Can you work these out from the drawing? Everything is in mm from the part's minimum corner. A direction names the side the tool comes from. Coordinates: 2 decimals unless noted, no trailing zeros. Order: outer loops, then holes, each group sorted by start corner. A loop starts at its lowest first (then second) coordinate and runs counter-clockwise, first axis right, second up. Notation, with made-up numbers: (30.5, -2) -> (48.5, -2) arc R6 cw to (48.5, 4) -> close; hole circle Ø10 at (-8.5, 67). An arc over 180 degrees is marked (long way). Answer in a Markdown table with one row per item.
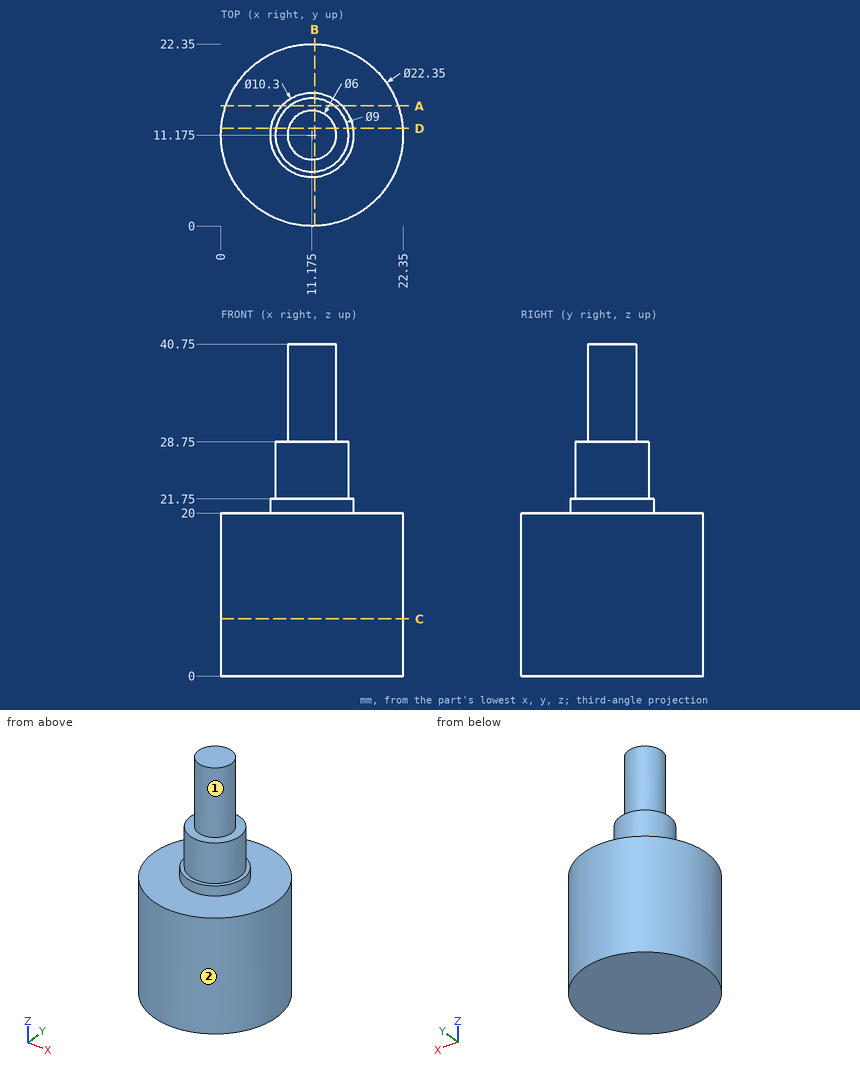
(1) Suppose I cut it at C-C (z = 7). Please give me the cut outline in (x, y) (3 decimals), and give its area (3 significant figures).
Response values:
| item | result |
|---|---|
| outline | circle Ø22.35 at (11.175, 11.175) |
| area | 392 mm2 |
(2) Suppose I cut it at A-A (y = 14.75). Please give me the cut outline in (x, z), and give its area (3 significant figures).
Response values:
| item | result |
|---|---|
| outline | (0.59, 0) -> (21.76, 0) -> (21.76, 20) -> (14.88, 20) -> (14.88, 21.75) -> (13.91, 21.75) -> (13.91, 28.75) -> (8.44, 28.75) -> (8.44, 21.75) -> (7.47, 21.75) -> (7.47, 20) -> (0.59, 20) -> close |
| area | 475 mm2 |
(3) Suppose I cut it at B-B (x = 11.5). Please give me the cut outline in (y, z).
Response values:
| item | result |
|---|---|
| outline | (0, 0) -> (22.35, 0) -> (22.35, 20) -> (16.31, 20) -> (16.31, 21.75) -> (15.66, 21.75) -> (15.66, 28.75) -> (14.16, 28.75) -> (14.16, 40.75) -> (8.19, 40.75) -> (8.19, 28.75) -> (6.69, 28.75) -> (6.69, 21.75) -> (6.04, 21.75) -> (6.04, 20) -> (0, 20) -> close |
(4) Will these pins go through, and if not, where does the flat tip stop? pin 1 Ø12 at (x, z) = (2.5, 7.5) entering from -Y; pin 2 Ø8 at (y, z) = (4, 34) entering from -X; pin 3 Ø10 at (x, y) = (20, 10.5) entering from +Z; pin 4 Ø8 at (x, z) = (10, 34) entering from +Y (3 decimals).
Response values:
| item | result |
|---|---|
| pin 1 | y = 0.32 |
| pin 2 | through |
| pin 3 | z = 28.75 |
| pin 4 | y = 14.175 |
(5) Suppose I cut it at D-D (y = 12). Please give me the cut outline in (x, z).
Response values:
| item | result |
|---|---|
| outline | (0.03, 0) -> (22.32, 0) -> (22.32, 20) -> (16.26, 20) -> (16.26, 21.75) -> (15.6, 21.75) -> (15.6, 28.75) -> (14.06, 28.75) -> (14.06, 40.75) -> (8.29, 40.75) -> (8.29, 28.75) -> (6.75, 28.75) -> (6.75, 21.75) -> (6.09, 21.75) -> (6.09, 20) -> (0.03, 20) -> close |
(6) On a 3-axis mill with a long thin cutter (end or side, diameter ignored), from which of +Z, -Z, +X, -X, +Y, -Y can I reach the whole of each face in a straight line? I mean the marked faces 1 and 2. Say none if no direction works.
Response values:
| item | result |
|---|---|
| face 1 | +Z |
| face 2 | +Z, -Z |
(7) I need wall thicknesses on line 1 (Z direction, x = 11, y = 15); line 2 (Z direction, x = 8.5, y = 15.5); line 3 (Y direction, x = 4, z = 5.5). Which ranges of each line are inside material? Lowest first, please. Write a range as [from, to].
Response values:
| item | result |
|---|---|
| line 1 | [0, 28.75] |
| line 2 | [0, 21.75] |
| line 3 | [2.61, 19.74] |
